```python
from build123d import *

# Parameters (mm, degrees)
F0_R      = 12.5
F1_DEPTH  = 30
F3_DEPTH  = 30.001
F4_R      = 4
F5_DEPTH  = 15
F6_W      = 3
F6_H      = 12.5
F7_DEPTH  = 30.001
F9_DEPTH  = 30
F10_W     = 20.1029244214
F10_H     = 2
F10_W_2   = 3
F10_W_3   = 20.1884878725
F11_DEPTH = 25.7
F12_R     = 2.65
F13_DEPTH = 17.001
F14_W     = 3
F14_H     = 0.5
F15_DEPTH = 2
F16_W     = 7.1528945421
F16_H     = 0.5
F17_DEPTH = 2


with BuildPart() as f1:
    # F0 (on Top) → F1 (new body)
    with BuildSketch(Plane.XY):
        Circle(F0_R)
    extrude(amount=F1_DEPTH)

    # F2 (on face) → F3 (cut, through all)
    with BuildSketch(Plane.XY.offset(30)):
        with BuildLine():
            ThreePointArc((-2.1028398647, 1.3520593565), (-0.7045922006, -2.3986558383), (2.5, 0))
            ThreePointArc((2.5, 0), (2.3986558383, 0.7045922006), (2.1028398647, 1.3520593565))
            Line((2.1028398647, 1.3520593565), (-2.1028398647, 1.3520593565))
        make_face()
    extrude(amount=-F3_DEPTH, mode=Mode.SUBTRACT)

    # F4 (on face) → F5 (cut)
    with BuildSketch(Plane.XY.offset(30)):
        Circle(F4_R)
        with BuildLine():
            ThreePointArc((2.1028398647, 1.3520593565), (2.3986558383, 0.7045922006), (2.5, 0))
            ThreePointArc((2.5, 0), (-0.7045922006, -2.3986558383), (-2.1028398647, 1.3520593565))
            Line((-2.1028398647, 1.3520593565), (2.1028398647, 1.3520593565))
        make_face(mode=Mode.SUBTRACT)
    extrude(amount=-F5_DEPTH, mode=Mode.SUBTRACT)

    # F6 (on face) → F7 (cut, through all)
    with BuildSketch(Plane.XY.offset(30)):
        with Locations((0, -6.25)):
            Rectangle(F6_W, F6_H)
    extrude(amount=-F7_DEPTH, mode=Mode.SUBTRACT)

    # F8 (on face) → F9 (join, through all)
    with BuildSketch(Plane.XY.offset(30)):
        with BuildLine():
            Line((-4.5, -21.6619037897), (-1.5, -21.6619037897))
            Line((-1.5, -21.6619037897), (-1.5, -12.409673646))
            ThreePointArc((-1.5, -12.409673646), (-3.0232085504, -12.1288997877), (-4.5, -11.6619037897))
            Line((-4.5, -11.6619037897), (-4.5, -21.6619037897))
        make_face()
        with BuildLine():
            Line((4.5, -21.6619037897), (4.5, -11.6619037897))
            ThreePointArc((4.5, -11.6619037897), (3.0232085504, -12.1288997877), (1.5, -12.409673646))
            Line((1.5, -12.409673646), (1.5, -21.6619037897))
            Line((1.5, -21.6619037897), (4.5, -21.6619037897))
        make_face()
    extrude(amount=-F9_DEPTH)

    # F10 (on face) → F11 (cut, symmetric)
    with BuildSketch(Plane.XZ.offset(21.6619037897)):
        with Locations((-8.5514622107, 16)):
            Rectangle(F10_W, F10_H)
        with Locations((3, 16)):
            Rectangle(F10_W_2, F10_H)
        with Locations((14.5942439362, 16)):
            Rectangle(F10_W_3, F10_H)
    extrude(amount=F11_DEPTH, both=True, mode=Mode.SUBTRACT)

    # F12 (on face) → F13 (cut, through all)
    with BuildSketch(Plane(origin=(-4.5, 0, 0), x_dir=(0, -1, 0), z_dir=(-1, 0, 0))):
        with Locations((16.6619037897, 23.5)):
            Circle(F12_R)
        with Locations((16.6619037897, 7.5)):
            Circle(F12_R)
    extrude(amount=-F13_DEPTH, mode=Mode.SUBTRACT)

    # F14 (on face) → F15 (join, through all)
    with BuildSketch(Plane.XY.offset(15)):
        with Locations((-3, -11.9119037897)):
            Rectangle(F14_W, F14_H)
        with Locations((3, -11.9119037897)):
            Rectangle(F14_W, F14_H)
    extrude(amount=F15_DEPTH)

    # F16 (on face) → F17 (join, through all)
    with BuildSketch(Plane.XY.offset(15)):
        with Locations((5.0764472711, -8.7709431903)):
            Rectangle(F16_W, F16_H)
        with Locations((-5.0764472711, -8.7709431903)):
            Rectangle(F16_W, F16_H)
    extrude(amount=F17_DEPTH)


solid = f1.part
```
Work out the finished part from the listing and answer in its coordinate system (mm). A direction names the side the tool comes from. Coordinates: 2 decimals unless noted, no trailing zeros. Write each loop counter-clockwise with the first axis right and the second up, starting at its lowest first coordinate (ties: lowest second). Pieces come first, ordered by that corner, then holes. Notation, with made-up numbers: (44, -8) - (68, -8) arc R8 cw to (68, 7) - close; hole circle Ø10 at (13, 4.25). An arc over 180 degrees is marked (long way). Answer as a JSON object with one key per item and string values.
Q1. Find section D-D (y = -11). Write down the section's boundary in (x, z), plus the area to 3 significant figures.
Results list:
{"outline": "(-5.94, 0) - (-1.5, 0) - (-1.5, 15) - (-5.94, 15) - close; (-5.94, 17) - (-1.5, 17) - (-1.5, 30) - (-5.94, 30) - close; (1.5, 0) - (5.94, 0) - (5.94, 15) - (1.5, 15) - close; (1.5, 17) - (5.94, 17) - (5.94, 30) - (1.5, 30) - close", "area": "248 mm^2"}
Q2. For a pull along X with two mould halves and no side action, classify faces 5 (the flat face through (-3, -4, 17)), 6 (the flat face through (1.5, -12, 15)), 7 (the cylindrical face through (0.49, 12.49, 14.79)) as pulls with the +X half, pulls with the -X half, needs draft (parallel to the pull), parting line crosses it, or undercut.
Results list:
{"face 5": "needs draft", "face 6": "undercut", "face 7": "parting line crosses it"}
Q3. Find section B-B (y = -18). State how many separate pieces and enclosed holes the cut face has, plus the area to 3 significant figures.
Results list:
{"separate pieces": "8", "enclosed holes": "0", "area": "113 mm^2"}
Q4. Which of the six approach directions +Z, -Z, +X, -X, +Y, -Y give full straight-line access (tool end or side, diameter ignored) to faces 1 (the flat face through (3, -21.662, 24)), 2 (the flat face through (4.5, -17, 19)), 3 (the flat face through (-4, -10, 15)), 4 (the flat face through (-3, -17, 17))?
Results list:
{"face 1": "+Z, -Z, +X, -X, -Y", "face 2": "+Z, -Z, +X, -Y", "face 3": "+X, -X", "face 4": "+X, -X, -Y"}
Q5. Consider L1, parallel to Z at x = -9, y = -7.5; L2, parallel to X at y = 0, z = 9; L3, parallel to X at y = -14, z = 18. Determine where each line is inside the solid, lowest interval first. Write a range as from..to.
Results list:
{"L1": "z = 0..15, 17..30", "L2": "x = -12.5..-2.5, 2.5..12.5", "L3": "x = -4.5..-1.5, 1.5..4.5"}
Q6. Find section C-C (x = 7). Write down the section's boundary in (y, z).
Results list:
{"outline": "(-10.36, 0) - (10.36, 0) - (10.36, 30) - (-10.36, 30) - (-10.36, 17) - (-9.02, 17) - (-9.02, 15) - (-10.36, 15) - close; hole (-8.52, 15) - (4.04, 15) - (4.04, 17) - (-8.52, 17) - close"}
Q7. Given pin 1 Ø1.6 at (x, z) = (6.5, 15.5) entering from -Y; pin 2 Ø0.6 at (x, z) = (3.5, 16) entering from -Y; pin 3 Ø3.5 at (x, y) = (2.5, -16) entering from -Z; pin 4 Ø4 at (y, z) = (-16, 24.5) entering from +X, each flat-ended and moving along its own axis, determine where each tip first touches the part or whether it passes through.
Results list:
{"pin 1": "stops at y = -11.03", "pin 2": "stops at y = -12.16", "pin 3": "stops at z = 0", "pin 4": "stops at x = 4.5"}
Q8. Find section A-A (z = 23.5). Write down the section's boundary in (x, y).
Results list:
{"outline": "(-4.5, -21.66) - (-1.5, -21.66) - (-1.5, -19.31) - (-4.5, -19.31) - close; (-4.5, -14.01) - (-1.5, -14.01) - (-1.5, -3.71) arc R4 cw (long way) to (1.5, -3.71) - (1.5, -14.01) - (4.5, -14.01) - (4.5, -11.66) arc R12.5 ccw (long way) to (-4.5, -11.66) - close; (1.5, -21.66) - (4.5, -21.66) - (4.5, -19.31) - (1.5, -19.31) - close"}
